```python
from build123d import *

# Parameters (mm, degrees)
F0_W     = 32
F0_H     = 30
F1_DEPTH = 2
F2_W     = 32
F2_H     = 27
F3_DEPTH = 2
F4_R     = 1.5
F5_DEPTH = 4.001
F6_R     = 3


with BuildPart() as f1:
    # F0 (on Front) → F1 (new body)
    with BuildSketch(Plane.XZ):
        Rectangle(F0_W, F0_H)
    extrude(amount=-F1_DEPTH)

    # F2 (on face) → F3 (join)
    with BuildSketch(Plane.XZ):
        with Locations((0, 1.5)):
            Rectangle(F2_W, F2_H)
    extrude(amount=F3_DEPTH)

    # F4 (on face) → F5 (cut, through all)
    with BuildSketch(Plane.XZ.offset(2)):
        with Locations((-11.5, 10.5)):
            Circle(F4_R)
        with Locations((11.5, 10.5)):
            Circle(F4_R)
    extrude(amount=-F5_DEPTH, mode=Mode.SUBTRACT)

    # F6
    f6_edges = [f1.edges().sort_by_distance(p)[0] for p in [
        (-16, 0, 15),
        (16, 0, 15),
    ]]
    fillet(f6_edges, radius=F6_R)


solid = f1.part
```
Here's how the part is built. I have some questions about the finished solid (model axes, mm). A direction names the side the tool comes from. Round coordinates to 2 decimals unless told otherwise and drop trailing zeros. Loops run counter-clockwise (first coordinate to the right, second up) from the corner with the lowest first, then second, coordinate; pieces in that order, holes last. Notation, with made-up numbers: (-4, 83) -> (35, 83) arc R31 cw to (35, 108) -> close; hole circle Ø10 at (20, 62.25). An arc over 180 degrees is marked (long way). Answer as CSV lines item,"result".
1. If we section it at B-B on x = -11.5: Please give me the cut outline in (y, z), plus the area to 3 significant figures.
Final values:
outline,"(-2, -12) -> (0, -12) -> (0, -15) -> (2, -15) -> (2, 9) -> (-2, 9) -> close; (-2, 12) -> (2, 12) -> (2, 15) -> (-2, 15) -> close"
area,"102 mm^2"
2. If we section it at D-D on x = 12: Please give me the cut outline in (y, z), plus the area to 3 significant figures.
Final values:
outline,"(-2, -12) -> (0, -12) -> (0, -15) -> (2, -15) -> (2, 9.09) -> (-2, 9.09) -> close; (-2, 11.91) -> (2, 11.91) -> (2, 15) -> (-2, 15) -> close"
area,"103 mm^2"
3. If we section it at C-C on x = -6.5: Please give me the cut outline in (y, z).
Final values:
outline,"(-2, -12) -> (0, -12) -> (0, -15) -> (2, -15) -> (2, 15) -> (-2, 15) -> close"
4. If we section it at A-A on y = -0.4: Please give me the cut outline in (x, z).
Final values:
outline,"(-16, -12) -> (16, -12) -> (16, 12) arc R3 ccw to (13, 15) -> (-13, 15) arc R3 ccw to (-16, 12) -> close; hole circle Ø3 at (-11.5, 10.5); hole circle Ø3 at (11.5, 10.5)"
5. Thinking about a two-plate mould opening in Z: for faces 1 (the face through (-16, 0, -2)), 2 (the face through (-13, -0.03, 10.57)), 3 (the face through (-15.14, 0.03, 14.1)), 4 (the face through (10, -0.03, 10.57)), which applies, released by +Z, released by -Z, zero draft, split by the parting line, or undercut?
Final values:
face 1,"zero draft"
face 2,"undercut"
face 3,"released by +Z"
face 4,"undercut"
6. For pin 1 (2.5 mm diameter, centred on x = -11.5, z = 10.5, fed in from +Y); pin 2 (0.9 mm diameter, centred on x = 3.5, z = -13, fed in from -Y); pin 3 (0.6 mm diameter, centred on x = 1, y = -1.5, fed in from -Z), each with a flat end and sliding along its axis, tell me the tip position at first contact or that it passes through.
Final values:
pin 1,"passes through"
pin 2,"stops at y = 0"
pin 3,"stops at z = -12"
7. If I drill on L1, parallel to X at y = -1.25, z = 10; L2, parallel to Z at x = 11.5, y = 0.7; L3, parallel to Z at x = 11, y = -1.2, over which ranges is the centre line in solid material (lowest first)?
Final values:
L1,"x = -16 to -12.91, -10.09 to 10.09, 12.91 to 16"
L2,"z = -15 to 9, 12 to 15"
L3,"z = -12 to 9.09, 11.91 to 15"
8. Which directions (+Z, -Z, +X, -X, +Y, -Y) give clear straight access to the entire face, cutting with the end or side of a thin tool? Please do faces 5 (the face through (0, 0, -13)), 6 (the face through (0, 0, 15)).
Final values:
face 5,"-Z, +X, -X, -Y"
face 6,"+Z, +X, -X, +Y, -Y"
